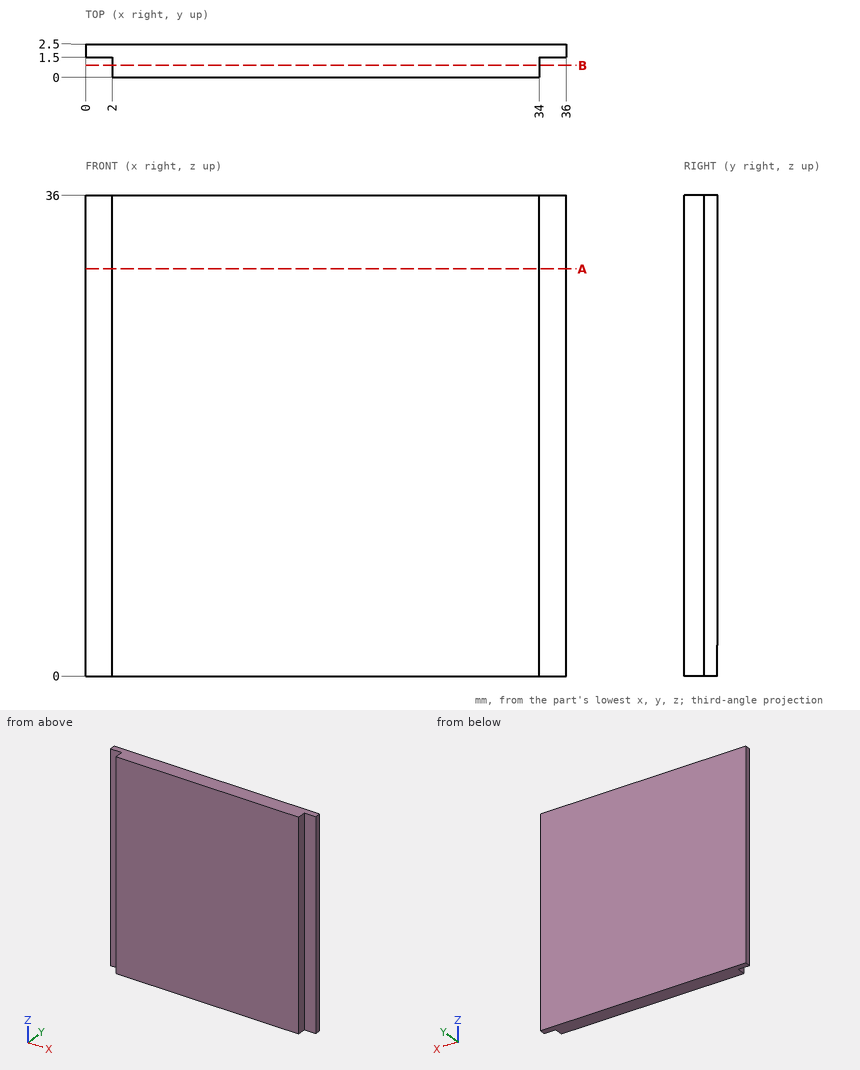
Study the drawing (mm; zero at the part's minimum x, y, z) and answer. Coordinates: 2 decimals unless noted, no trailing zeros. Write each loop counter-clockwise with the first axis right and the second up, starting at its lowest first coordinate (ties: lowest second). Pieces come first, ordered by that corner, then holes.
Q1. Each of these flat-tipped pins is pushed along its axis until it touches: pin 1 Ø1.6 at (x, z) = (35, 15) entering from -Y; pin 2 Ø0.5 at (y, z) = (0.5, 15) entering from -X; pin 3 Ø0.5 at (y, z) = (1, 13) entering from +X. Where does it stop, or does it pass through?
Q2. A cutting plane is placed at B-B, the plane y = 0.9. Give the vertices of the cut face in (x, z), then the cut area to 3 significant figures.
Q3. A cutting plane is placed at A-A, the plane z = 30.5. Give the vertices of the cut face in (x, y).
Q4. Find the intervals of material crossed by line 1 (X direction, y = 0.6, z = 32.5), in increasing order.
Findings below:
1. pin 1: stops at y = 1.5
1. pin 2: stops at x = 2
1. pin 3: stops at x = 34
2. outline: (2, 0) - (34, 0) - (34, 36) - (2, 36) - close
2. area: 1,150 mm2
3. outline: (0, 1.5) - (2, 1.5) - (2, 0) - (34, 0) - (34, 1.5) - (36, 1.5) - (36, 2.5) - (0, 2.5) - close
4. line 1: x = 2 to 34
